The model under review builds one solid part; all positions refer to its coordinate system, in mm. A direction names the side the tool comes from. Round coordinates to 2 decimals unless told otherwise and drop trailing zeros. Loops run counter-clockwise (first coordinate to the right, second up) from the corner with the lowest first, then second, coordinate; pieces in that order, holes last. Notation, with made-up numbers: M 31,33 L 72,33 A17 ccw 72,63 Z; hole C 9,-33 d11. An arc over 180 degrees is marked long. Return JSON: item names as keys, results as strings. Group by question number.
Q1. Consider section B-B (z = -7). State the section outline as (x, y) points.
Q2. Consider section A-A (y = 14). State the section outline as (x, z) points.
Q3. To check wall thickness, follow line 1 along X through (y, z) = (13.75, 2.5); line 2 along Y through (x, z) = (3.5, -8). State the ranges of each line that lie inside material, in increasing order.
Q4. Consider section C-C (x = 6.5). State the section outline as (y, z) points.
Q5. Clearance check with flat-ended pins moving along their axes: pin 1 Ø6.5 at (y, z) = (10.5, -1) entering from -X; pin 2 Ø5.5 at (x, z) = (-11.5, -1.5) entering from +Y; pin 3 Ø1 at (y, z) = (9.5, -5) entering from +X. State where each tip first meets the part, or that it passes through.
Q6. Draft analysis for pull direction X (two halves, no side actions). For faces 1 (the face through (-3.593, 9, -1)), 2 (the face through (-6.593, 9, -1)), 3 (the face through (-2, 0, -1)), state which applies: pulls with the +X half, pulls with the -X half, needs draft (parallel to the pull), parting line crosses it, or undercut.
Q7. For faces 4 (the face through (-0.193, 9, -1)), 5 (the face through (-5, 15, -1)), 6 (the face through (-10, 2, -1)), 7 (the face through (6, 2, -1)), list the 3-axis set-ups (+Z, -Z, +X, -X, +Y, -Y) from which the entire face can be reached by the end or side of a thin tool; tool diameter is ignored.
from build123d import *

# Parameters (mm, degrees)
ESQUISSE1_W             = 13
ESQUISSE1_H             = 20
BOSS_EXTRU_1_DEPTH      = 15
ESQUISSE2_W             = 2
ESQUISSE2_H             = 20
ESQUISSE2_W_2           = 3
ENL_V_MAT_EXTRU_2_DEPTH = 13
ESQUISSE4_W             = 20
ESQUISSE4_H             = 2
BOSS_EXTRU_2_DEPTH      = 5
ESQUISSE5_W             = 20
ESQUISSE5_H             = 2
BOSS_EXTRU_3_DEPTH      = 5
ESQUISSE6_W             = 20
ESQUISSE6_H             = 13
ENL_V_MAT_EXTRU_3_DEPTH = 0.2
ESQUISSE7_W             = 20
ESQUISSE7_H             = 13
ENL_V_MAT_EXTRU_4_DEPTH = 0.2
ESQUISSE8_W             = 20
ESQUISSE8_H             = 13
BOSS_EXTRU_4_DEPTH      = 0.2
ESQUISSE9_W             = 20
ESQUISSE9_H             = 13
BOSS_EXTRU_5_DEPTH      = 0.2


with BuildPart() as part:
    # Esquisse1 → Boss.-Extru.1 (new body)
    with BuildSketch(Plane(origin=(0, 0, 0), x_dir=(1, 0, 0), z_dir=(0, 1, 0))):
        with Locations((-1.892857143, 1.160714286)):
            Rectangle(ESQUISSE1_W, ESQUISSE1_H)
    extrude(amount=BOSS_EXTRU_1_DEPTH)

    # Esquisse2 → Enlèv. mat.-Extru.2 (cut)
    with BuildSketch(Plane(origin=(0, 15, 0), x_dir=(1, 0, 0), z_dir=(0, 1, 0))):
        with Locations((-7.392857143, 1.160714286)):
            Rectangle(ESQUISSE2_W, ESQUISSE2_H)
        with Locations((-1.892857143, 1.160714286)):
            Rectangle(ESQUISSE2_W_2, ESQUISSE2_H)
        with Locations((3.607142857, 1.160714286)):
            Rectangle(ESQUISSE2_W, ESQUISSE2_H)
    extrude(amount=-ENL_V_MAT_EXTRU_2_DEPTH, mode=Mode.SUBTRACT)

    # Esquisse4 → Boss.-Extru.2 (add)
    with BuildSketch(Plane.ZY.offset(8.392857143)):
        with Locations((-1.160714286, 1)):
            Rectangle(ESQUISSE4_W, ESQUISSE4_H)
    extrude(amount=BOSS_EXTRU_2_DEPTH)

    # Esquisse5 → Boss.-Extru.3 (add)
    with BuildSketch(Plane(origin=(4.607142857, 0, 0), x_dir=(0, 0, -1), z_dir=(1, 0, 0))):
        with Locations((1.160714286, 1)):
            Rectangle(ESQUISSE5_W, ESQUISSE5_H)
    extrude(amount=BOSS_EXTRU_3_DEPTH)

    # Esquisse6 → Enlèv. mat.-Extru.3 (cut)
    with BuildSketch(Plane.ZY.offset(0.392857143)):
        with Locations((-1.160714286, 8.5)):
            Rectangle(ESQUISSE6_W, ESQUISSE6_H)
    extrude(amount=-ENL_V_MAT_EXTRU_3_DEPTH, mode=Mode.SUBTRACT)

    # Esquisse7 → Enlèv. mat.-Extru.4 (cut)
    with BuildSketch(Plane(origin=(-3.392857143, 0, 0), x_dir=(0, 0, -1), z_dir=(1, 0, 0))):
        with Locations((1.160714286, 8.5)):
            Rectangle(ESQUISSE7_W, ESQUISSE7_H)
    extrude(amount=-ENL_V_MAT_EXTRU_4_DEPTH, mode=Mode.SUBTRACT)

    # Esquisse8 → Boss.-Extru.4 (add)
    with BuildSketch(Plane(origin=(2.607142857, 0, 0), x_dir=(0, 0, -1), z_dir=(1, 0, 0))):
        with Locations((1.160714286, 8.5)):
            Rectangle(ESQUISSE8_W, ESQUISSE8_H)
    extrude(amount=BOSS_EXTRU_4_DEPTH)

    # Esquisse9 → Boss.-Extru.5 (add)
    with BuildSketch(Plane.ZY.offset(6.392857143)):
        with Locations((-1.160714286, 8.5)):
            Rectangle(ESQUISSE9_W, ESQUISSE9_H)
    extrude(amount=BOSS_EXTRU_5_DEPTH)


solid = part.part
Values:
{
 "1": {"outline": "M -13.39,0 L 9.61,0 L 9.61,2 L 2.81,2 L 2.81,15 L -0.19,15 L -0.19,2 L -3.59,2 L -3.59,15 L -6.59,15 L -6.59,2 L -13.39,2 Z"},
 "2": {"outline": "M -6.59,-11.16 L -3.59,-11.16 L -3.59,8.84 L -6.59,8.84 Z; M -0.19,-11.16 L 2.81,-11.16 L 2.81,8.84 L -0.19,8.84 Z"},
 "3": {"line 1": "x = -6.59 to -3.59, -0.19 to 2.81", "line 2": "y = 0 to 2"},
 "4": {"outline": "M 0,-11.16 L 2,-11.16 L 2,8.84 L 0,8.84 Z"},
 "5": {"pin 1": "stops at x = -6.59", "pin 2": "stops at y = 2", "pin 3": "stops at x = 2.81"},
 "6": {"face 1": "undercut", "face 2": "pulls with the -X half", "face 3": "needs draft"},
 "7": {"face 4": "+Z, -Z, +Y", "face 5": "+Z, -Z, +X, -X, +Y", "face 6": "+Z, -Z, -X, +Y", "face 7": "+Z, -Z, +X, +Y"}
}
